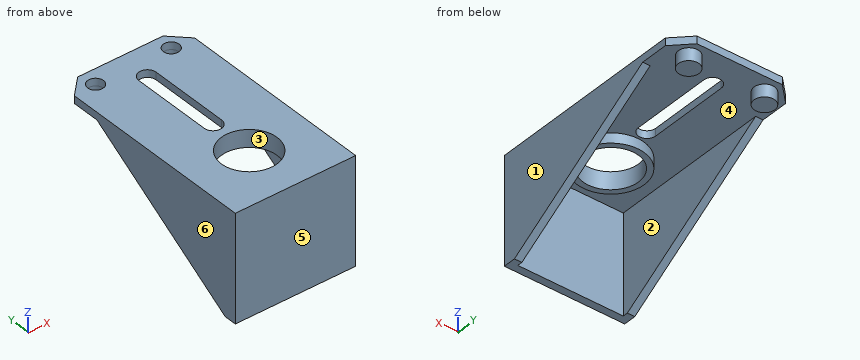
```python
from build123d import *
from OCP.BRepFilletAPI import BRepFilletAPI_MakeChamfer
from build123d.topology import SkipClean

# Parameters (mm, degrees)
SKETCH1_R                = 1.55
SKETCH1_R_2              = 1.5
SKETCH1_R_3              = 11
SKETCH1_R_4              = 3.175
BOSS_EXTRUDE1_DEPTH      = 3
BOSS_EXTRUDE2_START      = 3
SKETCH2_R                = 4.175
SKETCH2_R_2              = 3.175
BOSS_EXTRUDE2_DEPTH      = 3
BOSS_EXTRUDE3_START      = 2
SKETCH3_R                = 4.175
BOSS_EXTRUDE3_DEPTH      = 2
BOSS_EXTRUDE4_DEPTH      = 40
BOSS_EXTRUDE4_DEPTH_BACK = 3
SKETCH5_W                = 3
SKETCH5_H                = 5
BOSS_EXTRUDE5_DEPTH      = 3
BOSS_EXTRUDE7_DEPTH      = 3
BOSS_EXTRUDE9_DEPTH      = 3
BOSS_EXTRUDE10_START     = -3
SKETCH9_R                = 1.55
SKETCH9_R_2              = 1.5
SKETCH9_R_3              = 11
BOSS_EXTRUDE10_DEPTH     = 3
SKETCH10_R               = 11.2
CUT_EXTRUDE1_DEPTH       = 22.7
CUT_EXTRUDE2_DEPTH       = 10
SKETCH12_R               = 13.5
SKETCH12_R_2             = 11.2
BOSS_EXTRUDE11_DEPTH     = 4
SKETCH13_W               = 3
SKETCH13_H               = 76.55
BOSS_EXTRUDE13_DEPTH     = 3
BOSS_EXTRUDE14_DEPTH     = 3
BOSS_EXTRUDE15_DEPTH     = 3
SKETCH16_W               = 0.497079972
SKETCH16_H               = 40
CUT_EXTRUDE3_DEPTH       = 2
CHAMFER1_SIZE            = 3
CHAMFER1_SIZE_2          = 2.99439091
BOSS_EXTRUDE17_DEPTH     = 3


with BuildPart() as part:
    # Sketch1 → Boss-Extrude1 (new body)
    with BuildSketch(Plane.XY):
        Polygon((-33.421286346, -6), (-33.421286346, 36.5), (-33.421286346, 72.55), (-28.421286346, 77.55), (4.078713654, 77.55), (9.078713654, 72.55), (9.078713654, 36.5), (9.078713654, -6), align=None)
        with Locations((2.92772434, 30.5)):
            Circle(SKETCH1_R, mode=Mode.SUBTRACT)
        with Locations(Location((2.92772434, -0.5, 0), (0, 0, 180))):
            Circle(SKETCH1_R_2, mode=Mode.SUBTRACT)
        with Locations((-27.671286346, -0.5)):
            Circle(SKETCH1_R_2, mode=Mode.SUBTRACT)
        with Locations(Location((-28.07227566, 30.5, 0), (0, 0, 180))):
            Circle(SKETCH1_R_2, mode=Mode.SUBTRACT)
        with Locations((-12.171286346, 15.25)):
            Circle(SKETCH1_R_3, mode=Mode.SUBTRACT)
        with Locations((-27.421286346, 71.55)):
            Circle(SKETCH1_R_4, mode=Mode.SUBTRACT)
        with Locations(Location((3.078713654, 71.55, 0), (0, 0, 180))):
            Circle(SKETCH1_R_4, mode=Mode.SUBTRACT)
    extrude(amount=BOSS_EXTRUDE1_DEPTH)

    # Sketch2 → Boss-Extrude2 (add)
    # profile 1 of 2: a face of its own
    with SkipClean():  # the faces are left unmerged after this step: merging them gives an invalid solid
        with BuildSketch(Plane(origin=(0, 0, 0), x_dir=(-1, 0, 0), z_dir=(0, 0, -1)).offset(BOSS_EXTRUDE2_START)):
            with Locations((-3.078713654, 71.55)):
                Circle(SKETCH2_R)
            with Locations((-3.078713654, 71.55)):
                Circle(SKETCH2_R_2, mode=Mode.SUBTRACT)
        # profile 2 of 2: a face of its own
        with BuildSketch(Plane(origin=(0, 0, 0), x_dir=(-1, 0, 0), z_dir=(0, 0, -1)).offset(BOSS_EXTRUDE2_START)):
            with Locations((27.421286346, 71.55)):
                Circle(SKETCH2_R)
            with Locations((27.421286346, 71.55)):
                Circle(SKETCH2_R_2, mode=Mode.SUBTRACT)
        extrude(amount=-BOSS_EXTRUDE2_DEPTH)

    # Sketch3 → Boss-Extrude3 (add)
    with SkipClean():  # the faces are left unmerged after this step: merging them gives an invalid solid
        with BuildSketch(Plane(origin=(0, 0, -3), x_dir=(-1, 0, 0), z_dir=(0, 0, -1)).offset(BOSS_EXTRUDE3_START)):
            with Locations((-3.078713654, 71.55)):
                Circle(SKETCH3_R)
            with Locations((27.421286346, 71.55)):
                Circle(SKETCH3_R)
        extrude(amount=-BOSS_EXTRUDE3_DEPTH)

    # Sketch5 → Boss-Extrude5 (add)
    with SkipClean():  # the faces are left unmerged after this step: merging them gives an invalid solid
        with BuildSketch(Plane.XY.offset(3)):
            with Locations((10.578713654, 45.531399611)):
                Rectangle(SKETCH5_W, SKETCH5_H)
            with Locations((-34.921286346, 45.531399611)):
                Rectangle(SKETCH5_W, SKETCH5_H)
        extrude(amount=-BOSS_EXTRUDE5_DEPTH)



with BuildPart() as body_2:
    # Sketch4 → Boss-Extrude4 (new, two sides: drawn at the far end of the back side and taken through both)
    with BuildSketch(Plane(origin=(0, 0, 0), x_dir=(-1, 0, 0), z_dir=(0, 0, -1)).offset(-BOSS_EXTRUDE4_DEPTH_BACK)):
        Polygon((33.421286346, -6), (-9.078713654, -6), (-9.078713654, -4), (-12.078713654, -4), (-12.078713654, -9), (-9.078713654, -9), (33.259008686, -9), (36.259008686, -9), (36.259008686, -4), (33.259008686, -4), align=None)
    extrude(amount=BOSS_EXTRUDE4_DEPTH + BOSS_EXTRUDE4_DEPTH_BACK)


with BuildPart() as part_1:
    with SkipClean():  # the faces are left unmerged after this step: merging them gives an invalid solid
        add(part.part)

        add(body_2.part)  # Boss-Extrude7 merges body 2
        # Sketch6 → Boss-Extrude7 (add)
        with BuildSketch(Plane(origin=(9.078713654, 0, 0), x_dir=(0, 0, -1), z_dir=(1, 0, 0))):
            Polygon((0, 48.031399611), (40, -4), (36.156167209, -4), (0, 43.031399611), align=None)
        extrude(amount=BOSS_EXTRUDE7_DEPTH)

    # Sketch8 → Boss-Extrude9 (add)
    with BuildSketch(Plane.ZY.offset(36.421286346)):
        Polygon((0, 48.031399611), (0, 43.031399611), (-36.156167209, -4), (-40, -4), align=None)
    extrude(amount=-BOSS_EXTRUDE9_DEPTH)

    # Sketch9 → Boss-Extrude10 (add)
    with BuildSketch(Plane.XY.offset(3).offset(BOSS_EXTRUDE10_START)):
        with Locations((2.92772434, 30.5)):
            Circle(SKETCH9_R)
        with Locations((-28.07227566, 30.5)):
            Circle(SKETCH9_R_2)
        with Locations((-27.671286346, -0.5)):
            Circle(SKETCH9_R_2)
        with Locations((2.92772434, -0.5)):
            Circle(SKETCH9_R_2)
        with Locations((-12.171286346, 15.25)):
            Circle(SKETCH9_R_3)
    extrude(amount=BOSS_EXTRUDE10_DEPTH)

    # Sketch10 → Cut-Extrude1 (cut)
    with BuildSketch(Plane.XY.offset(3)):
        with Locations((-12.171286346, 14)):
            Circle(SKETCH10_R)
    extrude(amount=-CUT_EXTRUDE1_DEPTH, mode=Mode.SUBTRACT)

    # Sketch11 → Cut-Extrude2 (cut)
    with BuildSketch(Plane.XY.offset(3)):
        with BuildLine():
            Line((-8.671286346, 64.55), (-8.671286346, 32))
            ThreePointArc((-8.671286346, 32), (-12.171286346, 28.5), (-15.671286346, 32))
            Line((-15.671286346, 32), (-15.671286346, 64.55))
            ThreePointArc((-15.671286346, 64.55), (-12.171286346, 68.05), (-8.671286346, 64.55))
        make_face()
    extrude(amount=-CUT_EXTRUDE2_DEPTH, mode=Mode.SUBTRACT)

    # Sketch12 → Boss-Extrude11 (add)
    with BuildSketch(Plane(origin=(0, 0, 0), x_dir=(-1, 0, 0), z_dir=(0, 0, -1))):
        with Locations((12.171286346, 14)):
            Circle(SKETCH12_R)
        with Locations(Location((12.171286346, 14, 0), (0, 0, 180))):
            Circle(SKETCH12_R_2, mode=Mode.SUBTRACT)
    extrude(amount=BOSS_EXTRUDE11_DEPTH)

    # Sketch13 → Boss-Extrude13 (add)
    with BuildSketch(Plane.XY.offset(3)):
        with Locations((-34.921286346, 34.275)):
            Rectangle(SKETCH13_W, SKETCH13_H)
        Polygon((12.078713654, -4), (9.078713654, -4), (9.078713654, 72.55), (12.078713654, 72.555624881), align=None)
    extrude(amount=-BOSS_EXTRUDE13_DEPTH)

    # Sketch14 → Boss-Extrude14 (add)
    with BuildSketch(Plane(origin=(12.078713654, 0, 0), x_dir=(0, 0, -1), z_dir=(1, 0, 0))):
        Polygon((-3, 64.55), (-3, -9), (40, -9), (40, -4), align=None)
    extrude(amount=-BOSS_EXTRUDE14_DEPTH)

    # Sketch15 → Boss-Extrude15 (add)
    with BuildSketch(Plane.ZY.offset(36.421286346)):
        Polygon((3, 64.55), (-40, -4), (-40, -9), (3, -9), align=None)
    extrude(amount=-BOSS_EXTRUDE15_DEPTH)

    # Sketch16 → Cut-Extrude3 (cut)
    with BuildSketch(Plane(origin=(0, -4, 0), x_dir=(1, 0, 0), z_dir=(0, 1, 0))):
        with Locations((-33.17274636, 20)):
            Rectangle(SKETCH16_W, SKETCH16_H)
    extrude(amount=-CUT_EXTRUDE3_DEPTH, mode=Mode.SUBTRACT)

    # Chamfer1
    chamfer1_edges_1 = [part_1.edges().sort_by_distance(p)[0] for p in [
        (-36.421286346, 72.55, 1.5),
    ]]
    chamfer1_edges_2 = [part_1.edges().sort_by_distance(p)[0] for p in [
        (12.078713654, 72.555624881, 1.5),
    ]]
    chamfer1_side_2 = [part_1.faces().sort_by_distance(p)[0] for p in [
        (12.018825941, 72.555512593, 1.5),
    ]]
    chamfer1 = BRepFilletAPI_MakeChamfer(part_1.part.solid().wrapped)
    for e in chamfer1_edges_1:
        chamfer1.Add(CHAMFER1_SIZE - 0.0001, e.wrapped)
    for e in chamfer1_edges_2:
        chamfer1.Add(CHAMFER1_SIZE - 0.0001, CHAMFER1_SIZE_2 - 0.0001, e.wrapped, chamfer1_side_2[0].wrapped)
    add(Compound.cast(chamfer1.Shape()), mode=Mode.REPLACE)  # a hair under: the kernel refuses the full size

    # Sketch17 → Boss-Extrude17 (add)
    with BuildSketch(Plane.XY.offset(3)):
        Polygon((-33.421286346, 72.55), (-28.421286346, 77.55), (-12.171286346, 77.55), (-12.171286346, 78.05), (-29.370903561, 78.05), (-36.421286346, 70.999617215), (-36.421286346, 69.55), align=None)
        Polygon((-12.171286346, 78.05), (-12.171286346, 77.55), (4.078713654, 77.55), (9.078713654, 72.55), (12.078713654, 69.561233971), (12.078713654, 70.999617215), (5.028330869, 78.05), align=None)
    extrude(amount=-BOSS_EXTRUDE17_DEPTH)


solid = part_1.part
```
Work out the finished part from the listing and answer in its coordinate system (mm). Face numbers are marked on the shaded views. A direction names the side the tool comes from. Round coordinates to 2 decimals unless told otherwise and drop trailing zeros. Write each loop counter-clockwise with the first axis right and the second up, starting at its lowest first coordinate (ties: lowest second). Pieces come first, ordered by that corner, then holes. Notation, with made-up numbers: (52.5, 27.25) - (72.5, 27.25) arc R14 ccw to (72.5, 42.25) - close; hole circle Ø11 at (18.5, 9). An arc over 180 degrees is marked (long way). Return JSON: item names as keys, results as strings. Group by question number.
Q1. Each of these flat-tipped pins is pushed along its axis until it touches: pin 1 Ø8 at (x, y) = (-6, 8) entering from -Z; pin 2 Ø4 at (x, y) = (-27.42, 71.55) entering from +Z; pin 3 Ø4 at (x, y) = (1, 70.5) entering from -Z. Where does it stop, or does it pass through?
Q2. For the marked faces 1 and 2, determine the directions among +Z, -Z, +X, -X, +Y, -Y from which every point of the face is accessible in a straight line to the end or side of a thin tool.
Q3. The part is cut by section A-A on y = 62. Write down the section's boundary in (x, z).
Q4. The part is cut by section C-C on x = -14. Write down the section's boundary in (y, z).
Q5. Find the intervals of material crossed by L1, parallel to X at y = 71.55, z = 1.85; L2, parallel to X at y = -0.5, z = -31; L3, parallel to X at y = 71, z = 1, in increasing order.
Q6. The part is cut by section D-D on z = -26. Write down the section's boundary in (x, y), then the cut area to 3 significant figures.
Q7. The mould has two halves that part along Y. Classify the marked faces 3, 4, 5 and 6: released by +Y, released by -Y, zero draft, split by the parting line, or undercut.
Q8. The part is cut by section B-B on x = -19. Write down the section's boundary in (y, z), then the cut area to 3 significant figures.
Solved:
{
 "1": {"pin 1": "z = -4", "pin 2": "z = -3", "pin 3": "z = -5"},
 "2": {"face 1": "+Z, -Z, +X, +Y, -Y", "face 2": "-Z, +Y"},
 "3": {"outline": "(-36.42, 0) - (-15.67, 0) - (-15.67, 3) - (-36.42, 3) - close; (-8.67, 0) - (12.08, 0) - (12.08, 3) - (-8.67, 3) - close"},
 "4": {"outline": "(-9, -40) - (-6, -40) - (-6, 0) - (0.62, 0) - (0.62, -4) - (2.95, -4) - (2.95, 3) - (-9, 3) - close; (25.05, -4) - (27.38, -4) - (27.38, 0) - (29.02, 0) - (29.02, 3) - (25.05, 3) - close; (67.53, 0) - (78.05, 0) - (78.05, 3) - (67.53, 3) - close"},
 "5": {"L1": "-35.87 to -30.6, -24.25 to -0.1, 6.25 to 11.53", "L2": "-36.42 to -33.42, 9.08 to 12.08", "L3": "-36.42 to -30.55, -24.29 to -0.05, 6.21 to 12.08"},
 "6": {"outline": "(-36.42, -9) - (12.08, -9) - (12.08, 18.32) - (9.08, 18.32) - (9.08, -6) - (-33.42, -6) - (-33.42, 18.32) - (-36.42, 18.32) - close", "area": "291 mm²"},
 "7": {"face 3": "undercut", "face 4": "undercut", "face 5": "released by -Y", "face 6": "zero draft"},
 "8": {"outline": "(-9, -40) - (-6, -40) - (-6, 0) - (2.35, 0) - (2.35, -4) - (5.12, -4) - (5.12, 3) - (-9, 3) - close; (22.88, -4) - (25.65, -4) - (25.65, 0) - (78.05, 0) - (78.05, 3) - (22.88, 3) - close", "area": "350 mm²"}
}
